from build123d import *

# Parameters (mm, degrees)
SKETCH_1_W           = 40
SKETCH_1_H           = 64
SKETCH_1_R           = 3.2
EXTRUDE_1_DEPTH      = 4.2
SKETCH_2_R           = 16
SKETCH_2_W           = 20
SKETCH_2_H           = 20
EXTRUDE_2_DEPTH      = 10
EXTRUDE_2_DEPTH_BACK = 20
SKETCH_3_W           = 20
SKETCH_3_H           = 32
CUT_EXTRUDE_1_DEPTH  = 20
EXTRUDE_3_DEPTH      = 3
SKETCH_7_W           = 14
SKETCH_7_H           = 6
EXTRUDE_4_DEPTH      = 0.283766
EXTRUDE_5_DEPTH      = 3
SKETCH_9_W           = 6
SKETCH_9_H           = 14
EXTRUDE_6_DEPTH      = 1.612505
SKETCH_10_W          = 40
SKETCH_10_H          = 40
SKETCH_11_W          = 14
SKETCH_11_H          = 14
SKETCH_12_W          = 14
SKETCH_12_H          = 14
EXTRUDE_8_DEPTH      = 6
SKETCH_14_W          = 40
SKETCH_14_H          = 40
SKETCH_14_W_2        = 20
SKETCH_14_H_2        = 20
EXTRUDE_10_DEPTH     = 10
SKETCH_15_W          = 10
SKETCH_15_H          = 40
EXTRUDE_11_DEPTH     = 20
CUT_EXTRUDE_START    = -10
SKETCH_4_R           = 2
CUT_EXTRUDE_2_DEPTH  = 40
FILLET_2_R           = 5
FILLET_3_R           = 2


with BuildPart() as part:
    # Sketch 1 → Extrude 1 (new body)
    with BuildSketch(Plane.XY):
        Rectangle(SKETCH_1_W, SKETCH_1_H)
        with Locations((-12.5, 25)):
            Circle(SKETCH_1_R, mode=Mode.SUBTRACT)
        with Locations((12.5, 25)):
            Circle(SKETCH_1_R, mode=Mode.SUBTRACT)
        with Locations((12.5, -25)):
            Circle(SKETCH_1_R, mode=Mode.SUBTRACT)
        with Locations((-12.5, -25)):
            Circle(SKETCH_1_R, mode=Mode.SUBTRACT)
    extrude(amount=EXTRUDE_1_DEPTH)

    # Sketch 5 → Extrude 3 (add, symmetric)
    with BuildSketch(Plane(origin=(0, 0, 0), x_dir=(1, 0, 0), z_dir=(0, 1, 0))):
        Polygon((-20, -4.2), (-7, -33), (7, -33), (20, -4.2), align=None)
        Polygon((-13.805819277, -8.2), (-4, -8.2), (-4, -29.923661167), align=None, mode=Mode.SUBTRACT)
        Polygon((4, -29.923661167), (13.805819277, -8.2), (4, -8.2), align=None, mode=Mode.SUBTRACT)
    extrude(amount=EXTRUDE_3_DEPTH, both=True)



with BuildPart() as body_2:
    # Sketch 2 → Extrude 2 (new body, two sides)
    with BuildSketch(Plane(origin=(0, 0, 0), x_dir=(0, 0, -1), z_dir=(1, 0, 0))) as extrude_2_sk:
        with Locations((-49, 0)):
            Circle(SKETCH_2_R)
        with Locations((-49, 0)):
            Rectangle(SKETCH_2_W, SKETCH_2_H, mode=Mode.SUBTRACT)
    extrude(amount=EXTRUDE_2_DEPTH)
    extrude(extrude_2_sk.sketch, amount=-EXTRUDE_2_DEPTH_BACK)

    # Sketch 3 → Cut-Extrude 1 (cut)
    with BuildSketch(Plane.ZY.offset(20)):
        with Locations((49, 0)):
            Rectangle(SKETCH_3_W, SKETCH_3_H)
    extrude(amount=-CUT_EXTRUDE_1_DEPTH, mode=Mode.SUBTRACT)


with BuildPart() as part_1:
    add(part.part)

    add(body_2.part)  # Extrude 4 merges body 2
    # Sketch 7 → Extrude 4 (add)
    with BuildSketch(Plane.XY.offset(33)):
        Rectangle(SKETCH_7_W, SKETCH_7_H)
    extrude(amount=EXTRUDE_4_DEPTH)

    # Sketch 8 → Extrude 5 (add, symmetric)
    with BuildSketch(Plane(origin=(0, 0, 0), x_dir=(0, 0, -1), z_dir=(1, 0, 0))):
        Polygon((-4.2, 20), (-33, 7), (-33, -7), (-4.2, -20), align=None)
        Polygon((-8.2, 13.805819277), (-8.2, 4), (-29.923661167, 4), align=None, mode=Mode.SUBTRACT)
        Polygon((-8.2, -4), (-29.923661167, -4), (-8.2, -13.805819277), align=None, mode=Mode.SUBTRACT)
    extrude(amount=EXTRUDE_5_DEPTH, both=True)

    # Sketch 9 → Extrude 6 (add)
    with BuildSketch(Plane.XY.offset(33)):
        Rectangle(SKETCH_9_W, SKETCH_9_H)
    extrude(amount=EXTRUDE_6_DEPTH)

    # Sketch 10 → Loft 1 section 0
    with BuildSketch(Plane.XY.offset(4.2)):
        Rectangle(SKETCH_10_W, SKETCH_10_H)
    # Sketch 11 → Loft 1 section 1
    with BuildSketch(Plane.XY.offset(33)):
        Rectangle(SKETCH_11_W, SKETCH_11_H)
    loft()

    # Sketch 12 → Extrude 8 (add)
    with BuildSketch(Plane.XY.offset(33)):
        Rectangle(SKETCH_12_W, SKETCH_12_H)
    extrude(amount=EXTRUDE_8_DEPTH)

    # Sketch 14 → Extrude 10 (add)
    with BuildSketch(Plane(origin=(10, 0, 0), x_dir=(0, 0, -1), z_dir=(1, 0, 0))):
        with Locations((-49, 0)):
            Rectangle(SKETCH_14_W, SKETCH_14_H)
        with Locations((-49, 0)):
            Rectangle(SKETCH_14_W_2, SKETCH_14_H_2, mode=Mode.SUBTRACT)
    extrude(amount=-EXTRUDE_10_DEPTH)

    # Sketch 15 → Extrude 11 (add)
    with BuildSketch(Plane.ZY.offset(20)):
        with Locations((64, 0)):
            Rectangle(SKETCH_15_W, SKETCH_15_H)
        with Locations((34, 0)):
            Rectangle(SKETCH_15_W, SKETCH_15_H)
    extrude(amount=-EXTRUDE_11_DEPTH)

    # Sketch 4 → Cut-Extrude 2 (cut)
    with BuildSketch(Plane.XY.offset(39).offset(CUT_EXTRUDE_START)):
        with Locations((-12, 0)):
            Circle(SKETCH_4_R)
    extrude(amount=CUT_EXTRUDE_2_DEPTH, mode=Mode.SUBTRACT)

    # Fillet 2
    fillet_2_edges = [part_1.edges().sort_by_distance(p)[0] for p in [
        (-5, 20, 29),
        (-5, -20, 29),
        (-5, -20, 69),
        (-5, 20, 69),
    ]]
    fillet(fillet_2_edges, radius=FILLET_2_R)

    # Fillet 3
    fillet_3_edges = [part_1.edges().sort_by_distance(p)[0] for p in [
        (0, 15, 39),
        (0, -15, 39),
        (0, 15, 59),
        (0, -15, 59),
    ]]
    fillet(fillet_3_edges, radius=FILLET_3_R)


solid = part_1.part
Build history of the part. All positions in model axes, mm. A direction names the side the tool comes from. Round coordinates to 2 decimals unless told otherwise and drop trailing zeros. Write each loop counter-clockwise with the first axis right and the second up, starting at its lowest first coordinate (ties: lowest second). Pieces come first, ordered by that corner, then holes. Notation, with made-up numbers: (-6, 52.25) - (40, 52.25) arc R6 cw to (40, 56.25) - close; hole circle Ø1 at (-1.75, 87). An arc over 180 degrees is marked (long way). Use CSV: the item, a comma, the result in double quotes.
(1) Pin check, flat tips, straight feed: P1, Ø10, axis at x = -10.5, z = 32, coming from the +Y side; P2, Ø1.5, axis at x = -10, z = 13, coming from the -Y side; P3, Ø13, axis at x = 2.5, z = 44.5, coming from the -Y side; P4, Ø7.5, axis at x = -12.5, y = 25, coming from the -Z side. Stop position of each tip, or through.
Response:
P1,"y = 20"
P2,"y = -16.37"
P3,"y = -20"
P4,"z = 0"
(2) Band-saw the part on C-C (y = 0). Write the cut outline in (x, z), plus the area to 3 significant figures.
Response:
outline,"(-20, 0) - (20, 0) - (20, 4.2) - (8.81, 29) - (10, 29) - (10, 39) - (-10, 39) - (-10, 29) - (-8.81, 29) - (-20, 4.2) - close; (-20, 29) - (-14, 29) - (-14, 39) - (-20, 39) - close; (-20, 59) - (-14, 59) - (-14, 69) - (-20, 69) - close; (-10, 59) - (10, 59) - (10, 69) - (-10, 69) - close"
area,"1,400 mm²"
(3) 3-axis set-ups, long thin cutter, end or side, ignore diameter. For faces 1 (the flat face through (5, 10, 49)), 2 (the cylindrical face through (-5, 19, 31)), 3 (the cylindrical face through (-0.6, 14.93, 58.43)), 4 (the flat face through (10, 0, 63)), 5 (the flat face through (-0.28, -15.568, 14.018)): which of +Z, -Z, +X, -X, +Y, -Y reach the whole face in a straight line?
Response:
face 1,"+X, -X"
face 2,"+X, -X, +Y"
face 3,"-X, +Y, -Y"
face 4,"+Z, +X, +Y, -Y"
face 5,"+X, -X, -Y"
(4) Band-saw the part on A-A (y = 25). Write the cut outline in (x, z).
Response:
outline,"(-20, 0) - (-15.7, 0) - (-15.7, 4.2) - (-20, 4.2) - close; (-9.3, 0) - (9.3, 0) - (9.3, 4.2) - (-9.3, 4.2) - close; (15.7, 0) - (20, 0) - (20, 4.2) - (15.7, 4.2) - close"
(5) Wall check: line 1 (Y direction, x = -12.5, z = 2.5); line 2 (X direction, y = 0, z = 63.75); line 3 (Y direction, x = -12, z = 63). Give the ranges that are in metal, low to high.
Response:
line 1,"-32 to -28.2, -21.8 to 21.8, 28.2 to 32"
line 2,"-20 to -14, -10 to 10"
line 3,"-20 to -2, 2 to 20"
(6) Band-saw the part on D-D (x = 7). Write the cut outline in (y, z).
Response:
outline,"(-32, 0) - (32, 0) - (32, 4.2) - (20, 4.2) - (8.81, 29) - (15, 29) arc R5 ccw to (20, 34) - (20, 64) arc R5 ccw to (15, 69) - (-15, 69) arc R5 ccw to (-20, 64) - (-20, 34) arc R5 ccw to (-15, 29) - (-8.81, 29) - (-20, 4.2) - (-32, 4.2) - close; hole (-10, 39) - (10, 39) - (10, 59) - (-10, 59) - close"
(7) Mould opens along Z. For faces 6 (the flat face through (0, 26, 4.2)), 7 (the flat face through (1, -20, 49)), 8 (the flat face through (0.28, 15.568, 14.018)) say: pulls with the +Z half, pulls with the -Z half, needs draft (parallel to the pull), parting line crosses it, or undercut.
Response:
face 6,"pulls with the +Z half"
face 7,"needs draft"
face 8,"undercut"
(8) Band-saw the part on B-B (z = 44). Write the cut outline in (x, y), plus the area to 3 significant figures.
Response:
outline,"(0, -20) - (10, -20) - (10, -10) - (0, -10) - close; (0, 10) - (10, 10) - (10, 20) - (0, 20) - close"
area,"200 mm²"
